Geometry check sheet. Reference: the model listing, model coordinates, mm. Face numbers are marked on the shaded views. A direction names the side the tool comes from. Give positions to 0.01 mm unless a question says otherwise; leave off trailing zeros. Order: outer loops, then holes, each group sorted by start corner. A loop starts at its lowest first (then second) coordinate and runs counter-clockwise, first axis right, second up. Notation, with made-up numbers: M 29.5,47.5 L 60.5,47.5 A7 cw 60.5,59.5 Z; hole C -33,-12.75 d10. An arc over 180 degrees is marked long. Answer as CSV lines item,"result". Start each with the question number.
Q1. Section check C-C, the plane x = 45. Record the boundary of the cut face in (y, z).
Q2. Section check D-D, the plane x = 6. Record the boundary of the cut face in (y, z).
Q3. Thickness scan on line 1 (Y direction, x = 33, z = 0); line 2 (Y direction, x = 6, z = 0); line 3 (Z direction, x = 40, y = -11). Record the ranges inside material, lowest first.
Q4. Set-up check for the marked faces 4, 5 and 6: record each of +Z, -Z, +X, -X, +Y, -Y from which the full face is reachable in a straight line by a thin tool's end or side.
Q5. Mould release check, pull along Z, two halves, no side actions. Record for the marked faces 1, 2 and 3: +Z half, -Z half, draft (parallel to the pull), parting line (faces both ways), or undercut.
Q6. Go/stop test with flat-tipped pins: pin 1 (4 mm diameter, centred on y = 41, z = -62.5, fed in from +X); pin 2 (4 mm diameter, centred on x = 51, z = -54.5, fed in from -Y); pin 3 (1 mm diameter, centred on x = 4.5, z = -69.5, fed in from -Y). Record where each tip stops, or that it passes through.
```python
from build123d import *

# Parameters (mm, degrees)
FILLET1_R = 5
FILLET2_R = 5
FILLET3_R = 5


with BuildPart() as part:
    # Sketch1 → Revolve1 (revolve)
    with BuildSketch(Plane.XY, mode=Mode.PRIVATE) as revolve1_sk:
        Polygon((64.406730934, 20.074337298), (64.406730934, 35.087163878), (12.827354924, 44.181999517), (12.827354924, 79.50287687), (64.938484301, 90.726812428), (64.938484301, 100.877802998), (-64.938484301, 100.877802998), (-64.938484301, 90.726812428), (-12.827354924, 79.50287687), (-12.827354924, 44.181999517), (-64.406730934, 35.087163878), (-64.406730934, 20.074337298), align=None)
    revolve(revolve1_sk.sketch.rotate(Axis((-142.971560085, 0, 0), (1, 0, 0)), 90), axis=Axis((-142.971560085, 0, 0), (1, 0, 0)))

    # Fillet1
    fillet1_edges = [part.edges().sort_by_distance(p)[0] for p in [
        (-64.938484301, 0, -100.877802998),
    ]]
    fillet(fillet1_edges, radius=FILLET1_R)

    # Fillet2
    fillet2_edges = [part.edges().sort_by_distance(p)[0] for p in [
        (64.938484301, 0, -90.726812428),
        (64.938484301, 0, -100.877802998),
    ]]
    fillet(fillet2_edges, radius=FILLET2_R)

    # Fillet3
    fillet3_edges = [part.edges().sort_by_distance(p)[0] for p in [
        (-64.938484301, 0, -90.726812428),
    ]]
    fillet(fillet3_edges, radius=FILLET3_R)


solid = part.part
```
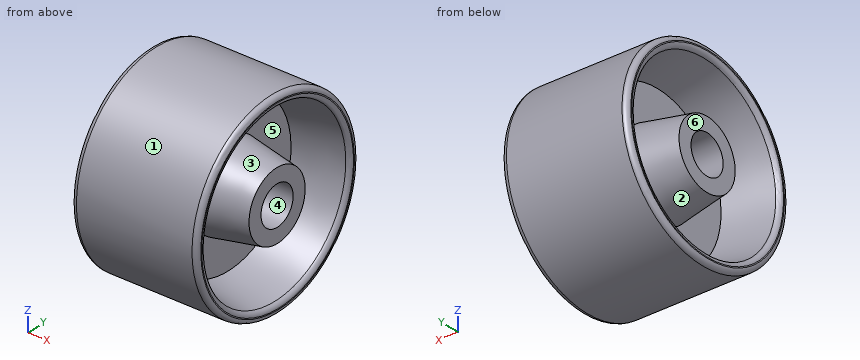
Answer block:
1,outline,"C 0,0 d201.76; C 0,0 d77.02; hole C 0,0 d172.86; hole C 0,0 d40.15"
2,outline,"C 0,0 d201.76; hole C 0,0 d40.15"
3,line 1,"y = -100.88 to -83.85, -40.63 to -20.07, 20.07 to 40.63, 83.85 to 100.88"
3,line 2,"y = -100.88 to -20.07, 20.07 to 100.88"
3,line 3,"z = -100.28 to -84.64, -37.82 to -16.79, 16.79 to 37.82, 84.64 to 100.28"
4,face 4,"+X, -X"
4,face 5,"+X"
4,face 6,"-X"
5,face 1,"parting line"
5,face 2,"undercut"
5,face 3,"undercut"
6,pin 1,"stops at x = 12.83"
6,pin 2,"stops at y = -86.14"
6,pin 3,"stops at y = -73.59"
